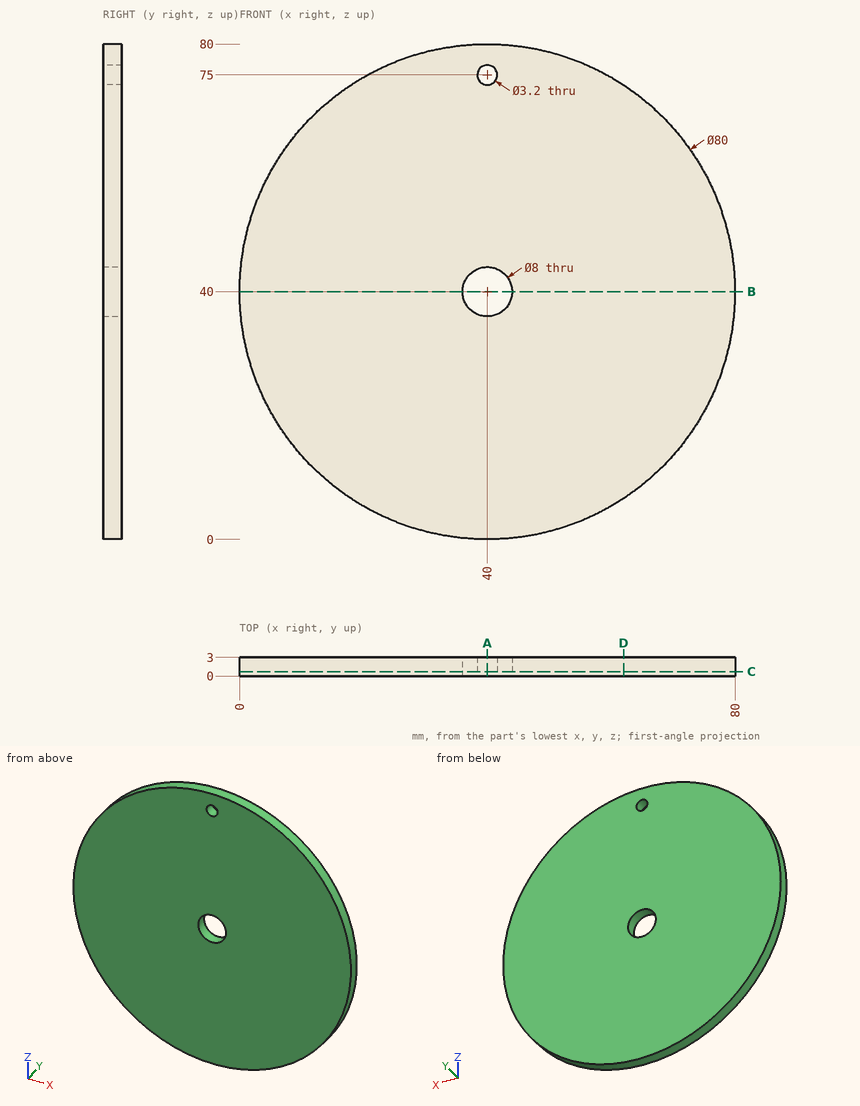
Can you work these out from the drawing? Everything is in mm from the part's minimum corner. Give positions to 0.01 mm unless a question says otherwise; leave off trailing zeros. Order: outer loops, then holes, each group sorted by start corner. A loop starts at its lowest first (then second) coordinate and runs counter-clockwise, first axis right, second up. Notation, with made-up numbers: (10, 75.5) -> (30, 75.5) arc R28 ccw to (30, 107.5) -> close; hole circle Ø2 at (-27, 29). An arc over 180 degrees is marked (long way). Return JSON: item names as keys, results as strings.
1. I need wall thicknesses on line 1 (Z direction, x = 40, y = 2); line 2 (X direction, y = 1.7, z = 75); line 3 (X direction, y = 1.95, z = 37). Which ranges of each line are inside material? Lowest first, please. Write a range as from..to.
Answer list:
{"line 1": "z = 0..36, 44..73.4, 76.6..80", "line 2": "x = 20.64..38.4, 41.6..59.36", "line 3": "x = 0.11..37.35, 42.65..79.89"}
2. Imagine slicing it at A-A on x = 40. List the corners of the cut face in (y, z) for me.
Answer list:
{"outline": "(0, 0) -> (3, 0) -> (3, 36) -> (0, 36) -> close; (0, 44) -> (3, 44) -> (3, 73.4) -> (0, 73.4) -> close; (0, 76.6) -> (3, 76.6) -> (3, 80) -> (0, 80) -> close"}
3. Imagine slicing it at B-B on z = 40. List the corners of the cut face in (x, y) for me.
Answer list:
{"outline": "(0, 0) -> (36, 0) -> (36, 3) -> (0, 3) -> close; (44, 0) -> (80, 0) -> (80, 3) -> (44, 3) -> close"}
4. Imagine slicing it at C-C on y = 0.7. List the corners of the cut face in (x, z) for me.
Answer list:
{"outline": "circle Ø80 at (40, 40); hole circle Ø8 at (40, 40); hole circle Ø3.2 at (40, 75)"}
5. Imagine slicing it at D-D on x = 62. List the corners of the cut face in (y, z) for me, then the cut area to 3 significant figures.
Answer list:
{"outline": "(0, 6.59) -> (3, 6.59) -> (3, 73.41) -> (0, 73.41) -> close", "area": "200 mm2"}
